Design review of the part shown in the three views and the two pictorial views. Dimensions are in mm from the part's minimum x, y and z. A direction names the side the tool comes from. Coordinates: 2 decimals unless noted, no trailing zeros. Write each loop counter-clockwise with the first axis right and the second up, starting at its lowest first coordinate (ties: lowest second). Pieces come first, ordered by that corner, then holes. Notation, with made-up numbers: (-36.75, 15) - (-3.75, 15) arc R18 ccw to (-3.75, 34) - close; hole circle Ø3 at (53.25, -23.5). An arc over 180 degrees is marked (long way). Return JSON: item names as keys, results as strings. Group by question number.
(1) We need section A-A on y = 26.65. State the section outline as (x, z) points.
(2) For pin 1 Ø1.5 at (x, y) = (13.5, 43) entering from +Z; pin 2 Ø5 at (y, z) = (20, 7) entering from -X, all flat-tipped, find the tip position at first contact; note any pin that passes through.
(3) To check wall thickness, follow L1, parallel to Y at x = 10, z = 0.95; L2, parallel to X at y = 33, z = 2.45; L3, parallel to X at y = 26.65, z = 1.55. State the ranges of each line that lie inside material, in increasing order. Write a range as from..to.
(4) Draft analysis for pull direction Y (two halves, no side actions). For the marked faces 3, 4, 5 and 6, state which applies: released by +Y, released by -Y, zero draft, split by the parting line, or undercut.
(5) We need section B-B on x = 3.65. State the section outline as (y, z) points, then the cut area to 3 significant figures.
(6) Tool access review of the marked faces 1 and 2: name each direction out of +Z, -Z, +X, -X, +Y, -Y from which nothing blocks a thin tool from reaching the whole face with its end or side.
(7) We need section D-D on x = 12.5. State the section outline as (y, z) points, then the cut area to 3 significant figures.
(8) We need section C-C on z = 13.75. State the section outline as (x, y) points, then the cut area to 3 significant figures.
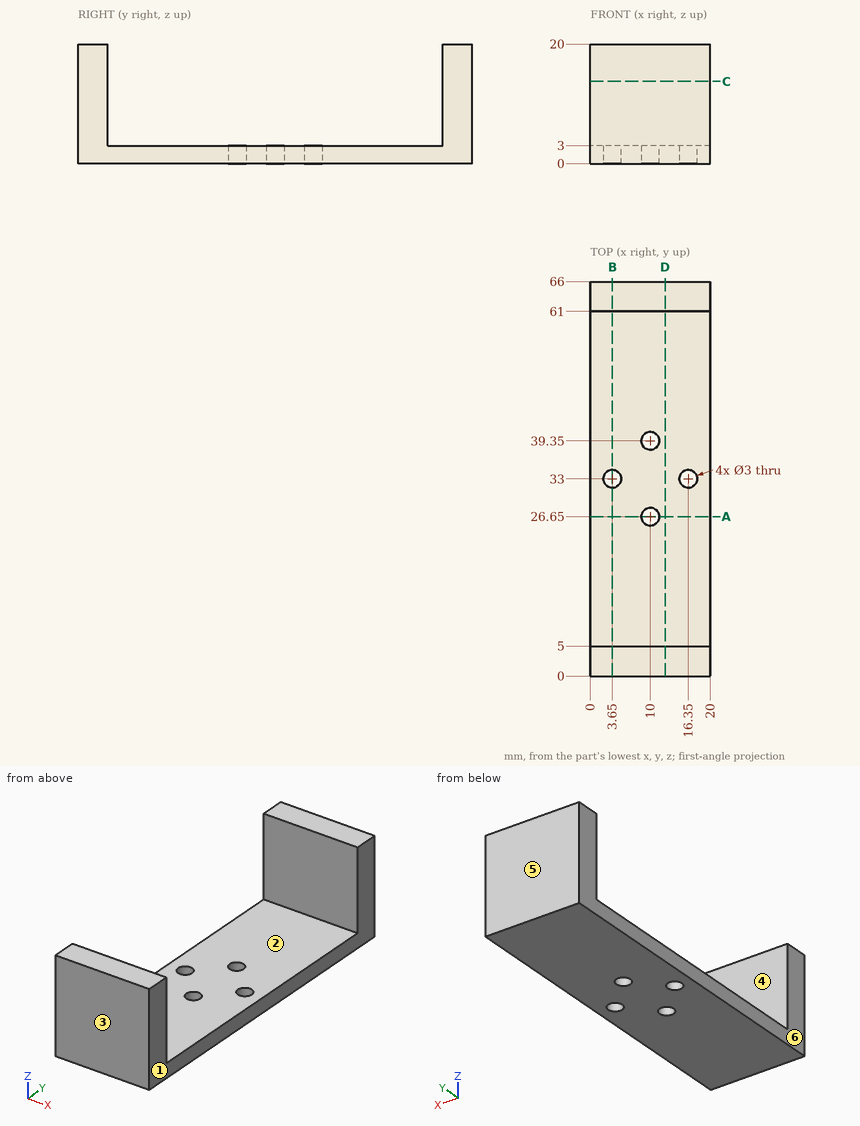
Ans:
{
 "1": {"outline": "(0, 0) - (8.5, 0) - (8.5, 3) - (0, 3) - close; (11.5, 0) - (20, 0) - (20, 3) - (11.5, 3) - close"},
 "2": {"pin 1": "z = 3", "pin 2": "through"},
 "3": {"L1": "0..25.15, 28.15..37.85, 40.85..66", "L2": "0..2.15, 5.15..14.85, 17.85..20", "L3": "0..8.5, 11.5..20"},
 "4": {"face 3": "released by -Y", "face 4": "undercut", "face 5": "released by +Y", "face 6": "zero draft"},
 "5": {"outline": "(0, 0) - (31.5, 0) - (31.5, 3) - (5, 3) - (5, 20) - (0, 20) - close; (34.5, 0) - (66, 0) - (66, 20) - (61, 20) - (61, 3) - (34.5, 3) - close", "area": "359 mm²"},
 "6": {"face 1": "+Z, -Z, +X, +Y, -Y", "face 2": "+Z, +X, -X"},
 "7": {"outline": "(0, 0) - (66, 0) - (66, 20) - (61, 20) - (61, 3) - (5, 3) - (5, 20) - (0, 20) - close", "area": "368 mm²"},
 "8": {"outline": "(0, 0) - (20, 0) - (20, 5) - (0, 5) - close; (0, 61) - (20, 61) - (20, 66) - (0, 66) - close", "area": "200 mm²"}
}
